Check sheet for the modelled part. Datum: model origin and axes. Units: mm. Face numbers are marked on the shaded views. A direction names the side the tool comes from. Give positions to 0.01 mm unless a question says otherwise; leave off trailing zeros. Write each loop counter-clockwise with the first axis right and the second up, starting at its lowest first coordinate (ties: lowest second). Pieces come first, ordered by that corner, then holes. Notation, with made-up numbers: M 34.5,77 L 80.5,77 A15 cw 80.5,87 Z; hole C 7,78.5 d4. An arc over 180 degrees is marked long. Write item = value, one per line. Start each with the question number.
1) Go/stop test with flat-tipped pins: pin 1 (4 mm diameter, centred on y = -3, z = -5.5, fed in from +X); pin 2 (7.5 mm diameter, centred on x = 25.5, y = -6.5, fed in from +Z); pin 3 (8 mm diameter, centred on y = -12.15, z = 16.91, fed in from -X); pin 4 (4 mm diameter, centred on x = 27.98, y = -12.14, fed in from -Z). Record where each tip stops, or that it passes through.
2) Mould release check, pull along Z, two halves, no side actions. Record for the marked faces 4, 5 and 6: released by +Z, released by -Z, zero draft, split by the parting line, or undercut.
3) Cross-section at B-B, the plane x = -7. Record the cut outline in (y, z).
4) Cross-section at C-C, the plane y = -2.5. Record the cut outline in (x, z).
5) Cross-section at D-D, the plane z = -22. Record the cut outline in (x, y).
6) Scan lines: line 1 along Y through (x, z) = (-10, 17); line 2 along Z through (x, y) = (-10.5, -10); line 3 along Z through (x, y) = (-7.5, -9.5). Record each from-to range of solid material in increasing order. Write a range as [from, to].
7) Access from +Z, -Z, +X, -X, +Y, -Y to the whole of each face (thin tool, end or side, straight path). Record for the marked faces 1, 2 and 3.
8) Cross-section at A-A, the plane z = 0. Record the cut outline in (x, y).
```python
from build123d import *

# Parameters (mm, degrees)
F1_W      = 70
F1_H      = 12
F2_DEPTH  = 24
F3_W      = 38
F3_H      = 50
F4_DEPTH  = 24
F5_R      = 12.5
F6_DEPTH  = 24
F7_W      = 4.3481588364
F7_H      = 18.8432261348
F8_DEPTH  = 24
F9_R      = 3.3
F10_DEPTH = 25
F11_R     = 3.3
F12_DEPTH = 25
F13_R     = 3
F14_DEPTH = 50
F15_R     = 5
F15_R_2   = 3
F16_DEPTH = 8
F17_SIZE  = 1
F18_SIZE  = 1


with BuildPart() as f2:
    # F1 (on Front) → F2 (new body)
    with BuildSketch(Plane.XZ):
        with Locations((0, -28.981200866)):
            Rectangle(F1_W, F1_H)
    extrude(amount=F2_DEPTH)

    # F3 (on Front) → F4 (join)
    with BuildSketch(Plane.XZ):
        Rectangle(F3_W, F3_H)
    extrude(amount=F4_DEPTH)

    # F5 (on face) → F6 (cut)
    with BuildSketch(Plane.XZ.offset(24)):
        Circle(F5_R)
    extrude(amount=-F6_DEPTH, mode=Mode.SUBTRACT)

    # F7 (on Front) → F8 (cut)
    with BuildSketch(Plane.XZ):
        with Locations((0, 19.3257555366)):
            Rectangle(F7_W, F7_H)
    extrude(amount=F8_DEPTH, mode=Mode.SUBTRACT)

    # F9 (on face) → F10 (cut)
    with BuildSketch(Plane(origin=(0, 0, -34.981200866), x_dir=(1, 0, 0), z_dir=(0, 0, -1))):
        with Locations((-28.0725006014, 12.1359182522)):
            Circle(F9_R)
    extrude(amount=-F10_DEPTH, mode=Mode.SUBTRACT)

    # F11 (on face) → F12 (cut)
    with BuildSketch(Plane(origin=(0, 0, -34.981200866), x_dir=(1, 0, 0), z_dir=(0, 0, -1))):
        with Locations((27.9758609831, 12.1359182522)):
            Circle(F11_R)
    extrude(amount=-F12_DEPTH, mode=Mode.SUBTRACT)

    # F13 (on face) → F14 (cut)
    with BuildSketch(Plane.YZ.offset(19)):
        with Locations((-12.1533777565, 16.9065129012)):
            Circle(F13_R)
    extrude(amount=-F14_DEPTH, mode=Mode.SUBTRACT)

    # F15 (on face) → F16 (cut)
    with BuildSketch(Plane.YZ.offset(19)):
        with Locations((-12.1533777565, 16.9065129012)):
            Circle(F15_R)
        with Locations((-12.1533777565, 16.9065129012)):
            Circle(F15_R_2, mode=Mode.SUBTRACT)
    extrude(amount=-F16_DEPTH, mode=Mode.SUBTRACT)

    # F17
    f17_edges = [f2.edges().sort_by_distance(p)[0] for p in [
        (19, 0, 1.0094),
        (19, -12, 25),
        (19, -24, 1.0094),
        (27, 0, -22.981201),
        (35, -12, -22.981201),
        (27, -24, -22.981201),
        (35, 0, -28.981201),
        (35, -24, -28.981201),
        (10.58704, -24, 25),
        (-10.58704, -24, 25),
        (-10.58704, 0, 25),
        (10.58704, 0, 25),
    ]]
    chamfer(f17_edges, length=F17_SIZE)

    # F18 (call 1 of 2: OpenCascade refuses the feature's edges together)
    f18_edges = [f2.edges().sort_by_distance(p)[0] for p in [
        (-19, -12, 25),
    ]]
    chamfer(f18_edges, length=F18_SIZE)

    # F18#2 (call 2 of 2)
    f18_2_edges = [f2.edges().sort_by_distance(p)[0] for p in [
        (-19, 0, 0.5094),
        (-19, -24, 0.5094),
        (-27, -24, -22.981201),
        (-35, -12, -22.981201),
        (-27, 0, -22.981201),
        (-35, 0, -28.981201),
        (-35, -24, -28.981201),
    ]]
    chamfer(f18_2_edges, length=F18_SIZE)


solid = f2.part
```
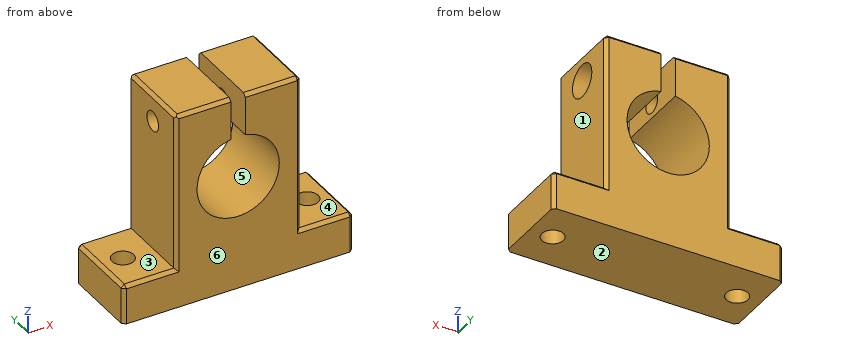
Reply:
q1.pin_1 = 19
q1.pin_2 = -22.98
q1.pin_3 = -19
q1.pin_4 = through
q2.face_4 = released by +Z
q2.face_5 = undercut
q2.face_6 = zero draft
q3.outline = M -24,-34.98 L 0,-34.98 L 0,-10.36 L -24,-10.36 Z; M -24,10.36 L 0,10.36 L 0,24 L -1,25 L -23,25 L -24,24 Z; hole C -12.15,16.91 d6
q4.outline = M -35,-34.98 L 35,-34.98 L 35,-23.98 L 34,-22.98 L 19,-22.98 L 19,24 L 18,25 L 2.17,25 L 2.17,12.31 A12.5 cw long -2.17,12.31 L -2.17,25 L -18,25 L -19,24 L -19,-22.98 L -34,-22.98 L -35,-23.98 Z
q5.outline = M -19,-23 L -18,-24 L 18,-24 L 19,-23 L 19,-1 L 18,0 L -18,0 L -19,-1 Z
q6.line_1 = [-24, -15.15], [-9.15, 0]
q6.line_2 = [-34.98, -6.78], [6.78, 14.82], [19, 25]
q6.line_3 = [-34.98, -10], [10, 15.51], [18.31, 25]
q7.face_1 = +Z, +X, +Y, -Y
q7.face_2 = -Z, +X, -X, +Y, -Y
q7.face_3 = +Z, -X, +Y, -Y
q8.outline = M -19,-23 L -18,-24 L -12.5,-24 L -12.5,0 L -18,0 L -19,-1 Z; M 12.5,-24 L 18,-24 L 19,-23 L 19,-1 L 18,0 L 12.5,0 Z
